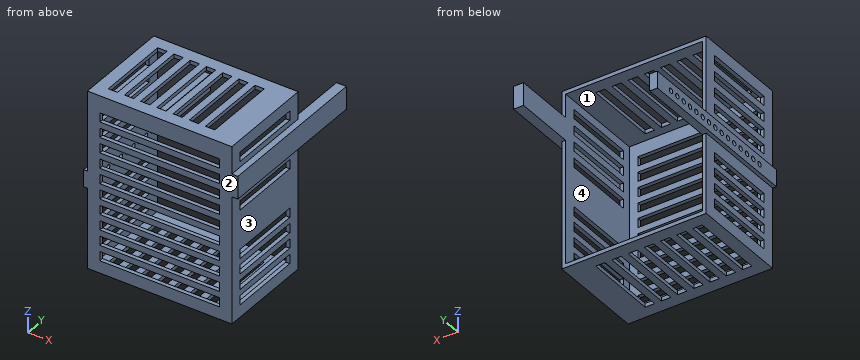
from build123d import *

# Parameters (mm, degrees)
SKETCH1_W           = 93.5
SKETCH1_H           = 115
BOSS_EXTRUDE1_DEPTH = 2.5
SKETCH2_W           = 93.5
SKETCH2_H           = 115
SKETCH2_W_2         = 88.5
SKETCH2_H_2         = 110
BOSS_EXTRUDE2_DEPTH = 60.5
SKETCH3_W           = 5
SKETCH3_H           = 11
BOSS_EXTRUDE3_DEPTH = 63
SKETCH4_W           = 5
SKETCH4_H           = 11
BOSS_EXTRUDE4_DEPTH = 50
SKETCH5_R           = 1.6
CUT_EXTRUDE1_DEPTH  = 5
LPATTERN1_COUNT     = 15
LPATTERN1_PITCH     = 6
SKETCH6_W           = 6
SKETCH6_H           = 47
CUT_EXTRUDE2_DEPTH  = 58.5
LPATTERN2_COUNT     = 7
LPATTERN2_PITCH     = 10.5
CUT_EXTRUDE3_START  = -50.25
SKETCH7_W           = 6
SKETCH7_H           = 47
CUT_EXTRUDE3_DEPTH  = 98
LPATTERN3_COUNT     = 4
LPATTERN3_PITCH     = 10.5
CUT_EXTRUDE4_START  = -50.25
SKETCH8_W           = 6
SKETCH8_H           = 47
CUT_EXTRUDE4_DEPTH  = 98
LPATTERN4_COUNT     = 4
LPATTERN4_PITCH     = 10
CUT_EXTRUDE5_START  = -3.5
SKETCH9_W           = 77.5
SKETCH9_H           = 6
CUT_EXTRUDE5_DEPTH  = 115
LPATTERN5_COUNT     = 10
LPATTERN5_PITCH     = 10
SKETCH11_W          = 6.441149118
SKETCH11_H          = 14.748011809
BOSS_EXTRUDE5_DEPTH = 40
SKETCH12_W          = 3.941149118
SKETCH12_H          = 14.748011809
BOSS_EXTRUDE6_DEPTH = 63


with BuildPart() as part:
    # Sketch1 → Boss-Extrude1 (new body)
    with BuildSketch(Plane(origin=(0, 0, 0), x_dir=(1, 0, 0), z_dir=(0, 1, 0))):
        Rectangle(SKETCH1_W, SKETCH1_H)
    extrude(amount=-BOSS_EXTRUDE1_DEPTH)

    # Sketch2 → Boss-Extrude2 (add)
    with BuildSketch(Plane(origin=(0, 0, 0), x_dir=(1, 0, 0), z_dir=(0, 1, 0))):
        Rectangle(SKETCH2_W, SKETCH2_H)
        Rectangle(SKETCH2_W_2, SKETCH2_H_2, mode=Mode.SUBTRACT)
    extrude(amount=BOSS_EXTRUDE2_DEPTH)

    # Sketch3 → Boss-Extrude3 (add, through all)
    with BuildSketch(Plane.XZ.offset(2.5)):
        with Locations((-46.75, 0)):
            Rectangle(SKETCH3_W, SKETCH3_H)
    extrude(amount=-BOSS_EXTRUDE3_DEPTH)

    # Sketch4 → Boss-Extrude4 (add)
    with BuildSketch(Plane(origin=(0, 60.5, 0), x_dir=(1, 0, 0), z_dir=(0, 1, 0))):
        with Locations((-46.75, 0)):
            Rectangle(SKETCH4_W, SKETCH4_H)
    extrude(amount=BOSS_EXTRUDE4_DEPTH)

    # Sketch5 → Cut-Extrude1 (cut)
    with BuildSketch(Plane.ZY.offset(49.25)):
        with Locations((0, 97.5)):
            Circle(SKETCH5_R)
    cut_extrude1 = extrude(amount=-CUT_EXTRUDE1_DEPTH, mode=Mode.SUBTRACT)

    # LPattern1: Cut-Extrude1 ×15
    with Locations(*[(0, -i * LPATTERN1_PITCH, 0) for i in range(1, LPATTERN1_COUNT)]):
        add(cut_extrude1, mode=Mode.SUBTRACT)

    # Sketch6 → Cut-Extrude2 (cut, symmetric)
    with BuildSketch(Plane.XY):
        with Locations((-35.75, 29)):
            Rectangle(SKETCH6_W, SKETCH6_H)
    cut_extrude2 = extrude(amount=CUT_EXTRUDE2_DEPTH, both=True, mode=Mode.SUBTRACT)

    # LPattern2: Cut-Extrude2 ×7
    with Locations(*[(i * LPATTERN2_PITCH, 0, 0) for i in range(1, LPATTERN2_COUNT)]):
        add(cut_extrude2, mode=Mode.SUBTRACT)

    # Sketch7 → Cut-Extrude3 (cut)
    with BuildSketch(Plane(origin=(0, 0, 0), x_dir=(0, 0, -1), z_dir=(1, 0, 0)).offset(CUT_EXTRUDE3_START)):
        with Locations((-46.5, 29)):
            Rectangle(SKETCH7_W, SKETCH7_H)
    cut_extrude3 = extrude(amount=CUT_EXTRUDE3_DEPTH, mode=Mode.SUBTRACT)

    # LPattern3: Cut-Extrude3 ×4
    with Locations(*[(0, 0, -i * LPATTERN3_PITCH) for i in range(1, LPATTERN3_COUNT)]):
        add(cut_extrude3, mode=Mode.SUBTRACT)

    # Sketch8 → Cut-Extrude4 (cut)
    with BuildSketch(Plane(origin=(0, 0, 0), x_dir=(0, 0, -1), z_dir=(1, 0, 0)).offset(CUT_EXTRUDE4_START)):
        with Locations((46.5, 29)):
            Rectangle(SKETCH8_W, SKETCH8_H)
    cut_extrude4 = extrude(amount=CUT_EXTRUDE4_DEPTH, mode=Mode.SUBTRACT)

    # LPattern4: Cut-Extrude4 ×4
    with Locations(*[(0, 0, i * LPATTERN4_PITCH) for i in range(1, LPATTERN4_COUNT)]):
        add(cut_extrude4, mode=Mode.SUBTRACT)

    # Sketch9 → Cut-Extrude5 (cut)
    with BuildSketch(Plane(origin=(0, 0, 0), x_dir=(1, 0, 0), z_dir=(0, 1, 0)).offset(CUT_EXTRUDE5_START)):
        with Locations((0, 46.5)):
            Rectangle(SKETCH9_W, SKETCH9_H)
    cut_extrude5 = extrude(amount=CUT_EXTRUDE5_DEPTH, mode=Mode.SUBTRACT)

    # LPattern5: Cut-Extrude5 ×10
    with Locations(*[(0, 0, i * LPATTERN5_PITCH) for i in range(1, LPATTERN5_COUNT)]):
        add(cut_extrude5, mode=Mode.SUBTRACT)

    # Sketch11 → Boss-Extrude5 (add)
    with BuildSketch(Plane(origin=(0, 60.5, 0), x_dir=(1, 0, 0), z_dir=(0, 1, 0))):
        with Locations((47.470574559, -32.398557857)):
            Rectangle(SKETCH11_W, SKETCH11_H)
    extrude(amount=BOSS_EXTRUDE5_DEPTH)

    # Sketch12 → Boss-Extrude6 (add, through all)
    with BuildSketch(Plane.XZ.offset(-60.5)):
        with Locations((48.720574559, 32.398557857)):
            Rectangle(SKETCH12_W, SKETCH12_H)
    extrude(amount=BOSS_EXTRUDE6_DEPTH)


solid = part.part
Work out the finished part from the listing and answer in its coordinate system (mm). Face numbers are marked on the shaded views. Coordinates: 2 decimals unless noted, no trailing zeros. Write each loop counter-clockwise with the first axis right and the second up, starting at its lowest first coordinate (ties: lowest second). Pieces come first, ordered by that corner, then holes. Notation, with made-up numbers: (28, -5.75) - (73, -5.75) arc R22 cw to (73, 25.25) - close; hole circle Ø8 at (63.25, -2). An arc over 180 degrees is marked (long way). One line per question, with ' | ' between items.
1) Consider probe 1 along Z at (x, y) = (35.5, 12); probe 2 along Z at (x, y) = (-46.9, 55.5); probe 3 along X at (y, z) = (48.5, 22). Determine where each line is inside the solid, lowest interval first. Write a range as [from, to].
Checks:
probe 1: [-57.5, -55], [55, 57.5] | probe 2: [-5.5, -1.6], [1.6, 5.5] | probe 3: [-46.75, -44.25], [44.25, 46.75]
2) Find section D-D, the plane y = 55.5. Determine the outline of the cut face in (x, z), and give its area (3 significant figures).
Checks:
outline: (-49.25, -5.5) - (-46.75, -5.5) - (-46.75, -57.5) - (46.75, -57.5) - (46.75, 25.02) - (50.69, 25.02) - (50.69, 39.77) - (46.75, 39.77) - (46.75, 57.5) - (-46.75, 57.5) - (-46.75, 5.5) - (-49.25, 5.5) - (-49.25, 1.6) - (-44.25, 1.6) - (-44.25, 55) - (44.25, 55) - (44.25, -55) - (-44.25, -55) - (-44.25, -1.6) - (-49.25, -1.6) - close | area: 1,090 mm2
3) Find section B-B, the plane z = 3.5. Determine the outline of the cut face in (x, y), and give its area (3 significant figures).
Checks:
outline: (-49.25, -2.5) - (-38.75, -2.5) - (-38.75, 0) - (-44.25, 0) - (-44.25, 110.5) - (-49.25, 110.5) - close; (38.75, -2.5) - (46.75, -2.5) - (46.75, 60.5) - (44.25, 60.5) - (44.25, 0) - (38.75, 0) - close | area: 750 mm2
4) Find section C-C, the plane x = -9.5. Give the number of separate pieces and of enclosed holes in the cut face, and give its area (3 significant figures).
Checks:
separate pieces: 11 | enclosed holes: 0 | area: 440 mm2
5) Find section A-A, the plane y = 73.5. Determine the outline of the cut face in (x, z), and give its area (3 significant figures).
Checks:
outline: (-49.25, -5.5) - (-44.25, -5.5) - (-44.25, -1.6) - (-49.25, -1.6) - close; (-49.25, 1.6) - (-44.25, 1.6) - (-44.25, 5.5) - (-49.25, 5.5) - close; (44.25, 25.02) - (50.69, 25.02) - (50.69, 39.77) - (44.25, 39.77) - close | area: 134 mm2
6) Flat-ended cylindrical pins translate along their axes: P1, Ø2, axis at x = 18, z = -56.5, coming from the +Y side; P2, Ø4, axis at x = 27.5, z = -42, coming from the +Y side; P3, Ø1.2, axis at y = -0.5, z = -6, coming from the -X side; P4, Ø0.8, axis at y = -1.5, z = -16.5, coming from the +X side. Find the tip coordinate at first contact, or state that the pin passes through.
Checks:
P1: y = 60.5 | P2: y = 0 | P3: x = -49.25 | P4: x = 46.75
7) The mould has two halves that part along X. Classify the marked faces 1, 2, 3 and 4: +X half, -X half, draft (parallel to the pull), parting line (faces both ways), or undercut.
Checks:
face 1: undercut | face 2: draft | face 3: +X half | face 4: undercut
